```python
from build123d import *

# Parameters (mm, degrees)
SKETCH_1_W      = 600
SKETCH_1_H      = 300
EXTRUDE_1_DEPTH = 200
SKETCH_2_R      = 25
EXTRUDE_2_DEPTH = 20
EXTRUDE_START   = 20
SKETCH_3_R      = 25
EXTRUDE_3_DEPTH = 20


with BuildPart() as part:
    # 草图1 → 凸台-拉伸1 (new body)
    with BuildSketch(Plane.XY):
        Rectangle(SKETCH_1_W, SKETCH_1_H)
    extrude(amount=EXTRUDE_1_DEPTH)

    # 草图2 → 凸台-拉伸2 (add)
    with BuildSketch(Plane.XZ.offset(150)):
        with Locations(Location((-200, 100, 0), (0, 0, 90))):
            Circle(SKETCH_2_R)
        with Locations(Location((200, 100, 0), (0, 0, 90))):
            Circle(SKETCH_2_R)
    extrude(amount=EXTRUDE_2_DEPTH)

    # 草图3 → 凸台-拉伸3 (add)
    with BuildSketch(Plane(origin=(0, 150, 0), x_dir=(1, 0, 0), z_dir=(0, 1, 0)).offset(EXTRUDE_START)):
        with Locations(Location((200, -100, 0), (0, 0, 270))):
            Circle(SKETCH_3_R)
        with Locations(Location((-200, -100, 0), (0, 0, 270))):
            Circle(SKETCH_3_R)
    extrude(amount=-EXTRUDE_3_DEPTH)


solid = part.part
```
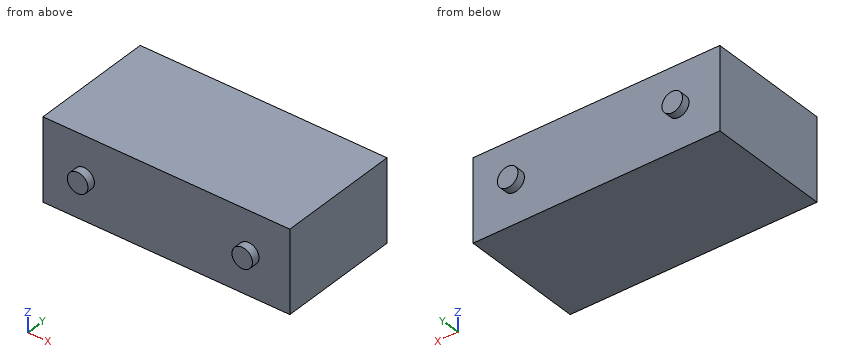
Work out the finished part from the listing and answer in its coordinate system (mm). Give positions to 0.01 mm unless a question says otherwise; leave off trailing zeros. Loops run counter-clockwise (first coordinate to the right, second up) from the corner with the lowest first, then second, coordinate; pieces in that order, holes last. Notation, with made-up numbers: M 22.25,65.5 L 77.25,65.5 A14 cw 77.25,86.5 Z; hole C -16,85.5 d4. An arc over 180 degrees is marked long. One line per item, written item: value. Start each with the question number.
1. Find section A-A (z = 100). Give the vertices of the cut face in (x, y).
2. Find the intervals of material crossed by probe 1 along Y at (x, z) = (-233, 139.5), in increasing order.
3. Find section D-D (x = 123). Give the vertices of the cut face in (y, z).
4. Find section C-C (z = 182.5). Give the vertices of the cut face in (x, y).
5. Each of these flat-tipped pins is pushed along its axis until it touches: P1, Ø4, axis at x = -50, y = 124.5, coming from the -Z side; P2, Ø12, axis at x = -22, z = 123.5, coming from the -Y side; P3, Ø3, axis at x = 165, z = 53.5, coming from the +Y side. Where does it stop, or does it pass through?
6. Find section B-B (x = 200). Give the vertices of the cut face in (y, z), and give its area (3 significant figures).
Reported:
1. outline: M -300,-150 L -225,-150 L -225,-170 L -175,-170 L -175,-150 L 175,-150 L 175,-170 L 225,-170 L 225,-150 L 300,-150 L 300,150 L 225,150 L 225,170 L 175,170 L 175,150 L -175,150 L -175,170 L -225,170 L -225,150 L -300,150 Z
2. probe 1: y = -150 to 150
3. outline: M -150,0 L 150,0 L 150,200 L -150,200 Z
4. outline: M -300,-150 L 300,-150 L 300,150 L -300,150 Z
5. P1: stops at z = 0
5. P2: stops at y = -150
5. P3: stops at y = 150
6. outline: M -170,75 L -150,75 L -150,0 L 150,0 L 150,75 L 170,75 L 170,125 L 150,125 L 150,200 L -150,200 L -150,125 L -170,125 Z
6. area: 62,000 mm²
